Geometry: see drawing. Coordinates: mm, zero at the bounding-box minimum. A direction names the side the tool comes from. Give positions to 0.01 mm unless a question says otherwise; leave off trailing zeros. Write each loop counter-clockwise with the first axis right and the second up, starting at its lowest first coordinate (ties: lowest second). Pieces come first, ordered by that corner, then holes. Notation, with made-up numbers: (64.25, -9.5) - (123.25, -9.5) arc R11 ccw to (123.25, -5.5) - close; hole circle Ø2 at (16, 87.25). An arc over 180 degrees is marked (long way). Return JSON: item names as keys, results as strings.
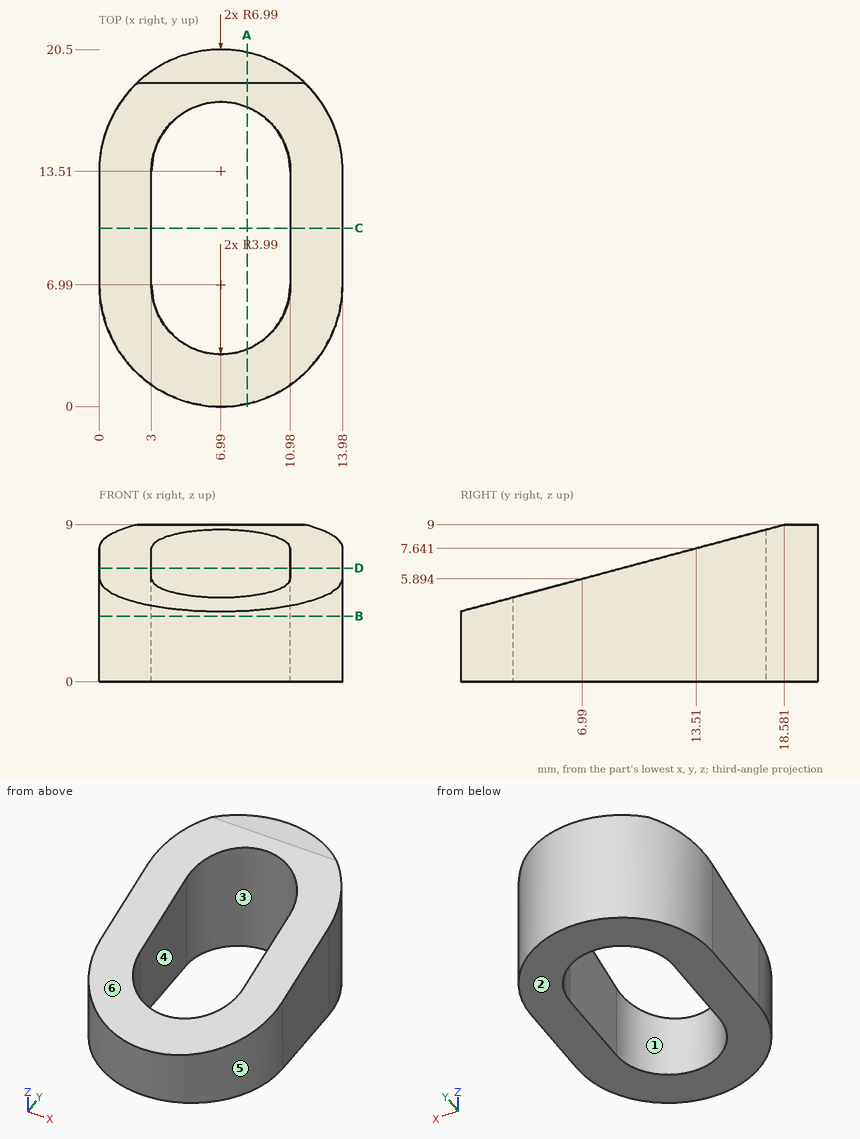
Q1. Material intervals for probe 1 along X at (y, z) = (7.75, 1); probe 2 along X at (y, z) = (17, 5.75) (1 decimal); probe 3 along Y at (x, z) = (5.25, 1.5), sorted ascending. Write a range as [from, to].
Answer key:
{"probe 1": "x = [0, 3], [10.98, 13.98]", "probe 2": "x = [0.9, 5.1], [8.9, 13]", "probe 3": "y = [0.22, 3.4], [17.1, 20.28]"}
Q2. Section query B-B, the plane z = 3.75. Return the cut outline in (x, y).
Answer key:
{"outline": "(0, 6.99) arc R6.99 ccw to (13.98, 6.99) - (13.98, 13.51) arc R6.99 ccw to (0, 13.51) - close; hole (3, 6.99) arc R3.99 ccw to (10.98, 6.99) - (10.98, 13.51) arc R3.99 ccw to (3, 13.51) - close"}
Q3. Mould query, pull axis X, two halves, no side actions, for the marked faces 3, 4, 5 and 6. Classes: pulls with the +X half, pulls with the -X half, needs draft (parallel to the pull), parting line crosses it, or undercut.
Answer key:
{"face 3": "undercut", "face 4": "undercut", "face 5": "parting line crosses it", "face 6": "needs draft"}
Q4. Section query A-A, the plane x = 8.5. Return the cut outline in (y, z) (1 decimal).
Answer key:
{"outline": "(0.2, 0) - (3.3, 0) - (3.3, 4.9) - (0.2, 4.1) - close; (17.2, 0) - (20.3, 0) - (20.3, 9) - (18.6, 9) - (17.2, 8.6) - close"}
Q5. Section query D-D, the plane z = 6.5. Return the cut outline in (x, y), plus the area to 3 significant figures.
Answer key:
{"outline": "(0, 9.25) - (3, 9.25) - (3, 13.51) arc R3.99 cw to (10.98, 13.51) - (10.98, 9.25) - (13.98, 9.25) - (13.98, 13.51) arc R6.99 ccw to (0, 13.51) - close", "area": "77.3 mm^2"}
Q6. Section query C-C, the plane y = 10.25. Return the cut outline in (x, z), plus the area to 3 significant figures.
Answer key:
{"outline": "(0, 0) - (3, 0) - (3, 6.77) - (0, 6.77) - close; (10.98, 0) - (13.98, 0) - (13.98, 6.77) - (10.98, 6.77) - close", "area": "40.6 mm^2"}
Q7. Pin query (flat end, axial travel): P1, Ø3, axis at x = 2.5, z = 4, coming from the -Y side; P2, Ø1, axis at x = 1.5, z = 2, coming from the +Y side (1 decimal); P3, Ø2, axis at x = 8.5, z = 6.5, coming from the +Y side. Return the tip coordinate at first contact, or that it passes through.
Answer key:
{"P1": "stops at y = 0.67", "P2": "stops at y = 18.4", "P3": "stops at y = 20.48"}
Q8. Set-up query: the marked faces 1 and 2. Return all of +Z, -Z, +X, -X, +Y, -Y with unobstructed straight access to the full face (end or side cutting, diameter ignored); none if empty.
Answer key:
{"face 1": "+Z, -Z", "face 2": "-Z, +X, -X, +Y, -Y"}
